Here's how the part is built. I have some questions about the finished solid (model axes, mm). Round coordinates to 2 decimals unless told otherwise and drop trailing zeros. Order: outer loops, then holes, each group sorted by start corner. A loop starts at its lowest first (then second) coordinate and runs counter-clockwise, first axis right, second up.
Autodesk Inventor part; units mm, degrees
ref_plane "YZ Plane" through (0, 0, 0) normal (1, 0, 0) x (0, 1, 0)
ref_plane "XZ Plane" through (0, 0, 0) normal (0, 1, 0) x (-1, 0, 0)
ref_plane "XY Plane" through (0, 0, 0) normal (0, 0, 1) x (1, 0, 0)
sketch "Skizze1" plane through (0, 0, 0) normal (0, 0, 1) x (1, 0, 0)
  line L0 (-56, 0) -> (56, 0)
  line L1 (0, -7.7) -> (0, 7.7)
  line L2 (-40, 5.5) -> (40, 5.5)
  line L3 (40, 5.5) -> (40, -5.5)
  line L4 (40, -5.5) -> (-40, -5.5)
  line L5 (-40, -5.5) -> (-40, 5.5)
  point P0 (0, 0)
  dimension "d0" = 11
  dimension "d1" = 80
extrude "Extrusion1" add sketch "Skizze1" along normal blind 1
sketch "Skizze2" plane through (0, 0, 1) normal (0, 0, 1) x (1, 0, 0)
  line L0 (-140, 0) -> (140, 0)
  line L1 (0, -7.7) -> (0, 7.7)
  point P0 (0, 0)
  point P1 (-30, 0)
  point P2 (30, 0)
  dimension "d4" = 60
hole "Bohrung1" at (-30, 0, 1) at (30, 0, 1) direction (0, 0, -1) diameter 2.4 end through all countersink diameter 4.5 countersink angle 90
sketch "Skizze3" plane through (40, -5.5, 0) normal (1, 0, 0) x (0, 0, -1)
  line L0 (0, 11) -> (0, 0)
  line L1 (0, 11) -> (-1, 11)
  line L2 (-1, 0) -> (-1, 11)
  line L3 (0, 0) -> (-1, 0)
  point P0 (0, 5.5)
extrude "Extrusion2" add sketch "Skizze3" along normal blind 6.5
fillet "Rundung1" radius 5 2 edges at (46.5, -5.5, 0.5) (46.5, 5.5, 0.5)
properties part number "13_1087_041"
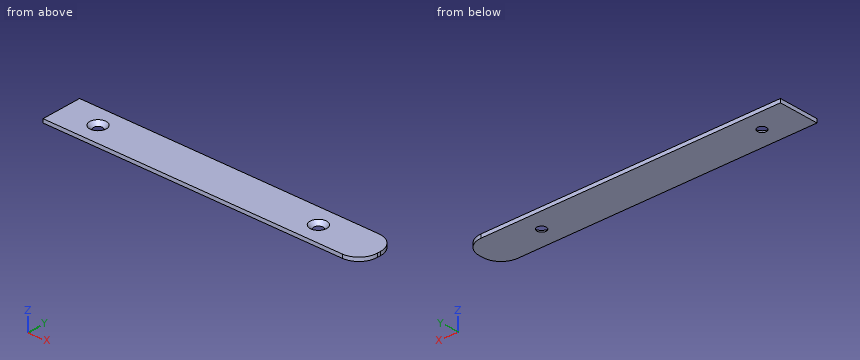
1. If we section it at B-B, the plane x = 30: Write out the boundary of the cut face in (y, z), and give its area (3 significant figures).
Evaluation:
outline: (-5.5, 0) - (-1.25, 0) - (-2.25, 1) - (-5.5, 1) - close; (1.25, 0) - (5.5, 0) - (5.5, 1) - (2.25, 1) - close
area: 7.50 mm2
2. If we section it at D-D, the plane y = 4.75: Write out the boundary of the cut face in (x, z), and give its area (3 significant figures).
Evaluation:
outline: (-40, 0) - (44.13, 0) - (44.13, 1) - (-40, 1) - close
area: 84.1 mm2
3. If we section it at A-A, the plane z = 0.35: Write out the boundary of the cut face in (x, y).
Evaluation:
outline: (-40, -5.5) - (41.5, -5.5) arc R5 ccw to (46.5, -0.5) - (46.5, 0.5) arc R5 ccw to (41.5, 5.5) - (-40, 5.5) - close; hole circle Ø3.2 at (-30, 0); hole circle Ø3.2 at (30, 0)
4. I need wall thicknesses on probe 1 along X at (y, z) = (0, 0.15); probe 2 along X at (y, z) = (1, 0.25); probe 3 along Y at (x, z) = (-29.5, 0.9). Which ranges of each line are inside material? Lowest first, please.
Evaluation:
probe 1: x = -40 to -31.4, -28.6 to 28.6, 31.4 to 46.5
probe 2: x = -40 to -31.12, -28.88 to 28.88, 31.12 to 46.47
probe 3: y = -5.5 to -2.09, 2.09 to 5.5
5. If we section it at C-C, the plane y = -4.5: Write out the boundary of the cut face in (x, z), and give its area (3 significant figures).
Evaluation:
outline: (-40, 0) - (44.5, 0) - (44.5, 1) - (-40, 1) - close
area: 84.5 mm2
